Work out the finished part from the listing and answer in its coordinate system (mm). Face numbers are marked on the shaded views. Round coordinates to 2 decimals unless told otherwise and drop trailing zeros. Write each loop counter-clockwise with the first axis right and the second up, starting at its lowest first coordinate (ties: lowest second). Pieces come first, ordered by that corner, then holes. Notation, with made-up numbers: M 64,-27 L 72,-27 A27 cw 72,7 Z; hole C 69.5,38 d6. An arc over 180 degrees is marked long. Answer in a Markdown table with one row per item.
```python
from build123d import *

# Parameters (mm, degrees)
F0_R     = 22.25
F0_R_2   = 20
F1_DEPTH = 50
F0_R_3   = 24.75
F2_DEPTH = 2
F3_R     = 1.99999


# Not quite as in the source:
# - a fillet or chamfer is up to 0.001 mm smaller than in the source, because OpenCascade refuses the exact size


with BuildPart() as f1:
    # F0 (on Top) → F1 (new body)
    with BuildSketch(Plane.XY):
        Circle(F0_R)
        Circle(F0_R_2, mode=Mode.SUBTRACT)
    extrude(amount=F1_DEPTH)

    # F0 (on Top) → F2 (join)
    with BuildSketch(Plane.XY):
        Circle(F0_R_3)
        Circle(F0_R, mode=Mode.SUBTRACT)
    extrude(amount=F2_DEPTH)

    # F3 (radius 2 in the source; OpenCascade refuses exactly that, so slightly less here)
    f3_edges = [f1.edges().sort_by_distance(p)[0] for p in [
        (-24.75, 0, 0),
    ]]
    fillet(f3_edges, radius=F3_R)


solid = f1.part
```
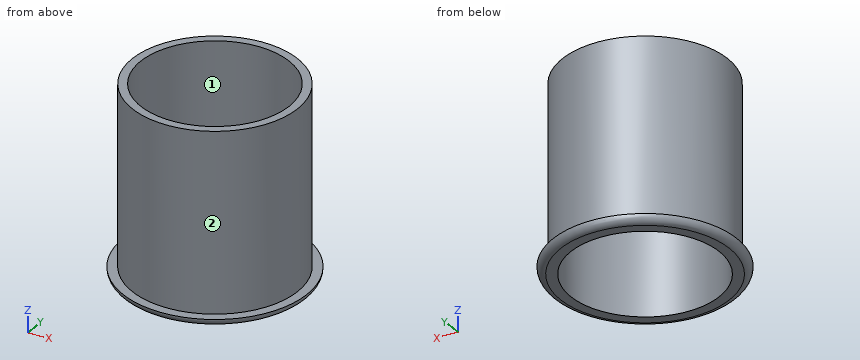
1. Given pin 1 (3 mm diameter, centred on y = 9, z = 10.5, fed in from +X); pin 2 (6 mm diameter, centred on y = -5, z = 18.5, fed in from +X); pin 3 (5 mm diameter, centred on x = -6.5, z = 40, fed in from +Y), each flat-ended and moving along its own axis, determine where each tip first touches the part or whether it passes through.
Calculated:
| item | result |
|---|---|
| pin 1 | stops at x = 20.95 |
| pin 2 | stops at x = 22.16 |
| pin 3 | stops at y = 21.89 |
2. The part is cut by section C-C (z = 35). Determine the outline of the cut face in (x, y), plus the area to 3 significant figures.
Calculated:
| item | result |
|---|---|
| outline | C 0,0 d44.5; hole C 0,0 d40 |
| area | 299 mm² |
3. Determine the mould class of the marked faces 1 and 2 for opening direction Y: released by +Y, released by -Y, zero draft, split by the parting line, or undercut.
Calculated:
| item | result |
|---|---|
| face 1 | undercut |
| face 2 | split by the parting line |
4. Consider line 1 along Y through (x, z) = (-0.5, 10.5); line 2 along X through (y, z) = (13.5, 10); line 3 along Y through (x, z) = (-14, 28). Determine where each line is inside the solid, lowest interval first. Write a range as from..to.
Calculated:
| item | result |
|---|---|
| line 1 | y = -22.24..-19.99, 19.99..22.24 |
| line 2 | x = -17.69..-14.76, 14.76..17.69 |
| line 3 | y = -17.29..-14.28, 14.28..17.29 |
